from build123d import *

# Parameters (mm, degrees)
BOSS_EXTRUDE1_DEPTH     = 1.6
CUT_EXTRUDE1_DEPTH      = 56.62202801
CUT_EXTRUDE1_DEPTH_BACK = 56.62202801
SKETCH3_R               = 1.5
SKETCH4_W               = 24
SKETCH4_H               = 10
SKETCH4_W_2             = 12
BOSS_EXTRUDE2_DEPTH     = 14
SKETCH5_W               = 18
SKETCH5_H               = 61
BOSS_EXTRUDE3_DEPTH     = 13.56


with BuildPart() as part:
    # Sketch2 → Boss-Extrude1 (new body)
    with BuildSketch(Plane(origin=(0, 0, 0), x_dir=(1, 0, 0), z_dir=(0, 1, 0))):
        with BuildLine():
            Line((34, 41.5), (-34, 41.5))
            ThreePointArc((-34, 41.5), (-36.121320344, 40.621320344), (-37, 38.5))
            Line((-37, 38.5), (-37, -38.5))
            ThreePointArc((-37, -38.5), (-36.121320344, -40.621320344), (-34, -41.5))
            Line((-34, -41.5), (34, -41.5))
            ThreePointArc((34, -41.5), (36.121320344, -40.621320344), (37, -38.5))
            Line((37, -38.5), (37, 38.5))
            ThreePointArc((37, 38.5), (36.121320344, 40.621320344), (34, 41.5))
        make_face()
    extrude(amount=BOSS_EXTRUDE1_DEPTH)

    # Sketch3 → Cut-Extrude1 (cut, two sides: drawn at the far end of the back side and taken through both)
    with BuildSketch(Plane(origin=(0, 1.6, 0), x_dir=(1, 0, 0), z_dir=(0, 1, 0)).offset(-CUT_EXTRUDE1_DEPTH_BACK)):
        with Locations(Location((-33, 23.5, 0), (0, 0, 270))):
            Circle(SKETCH3_R)
        with Locations(Location((33, 23.5, 0), (0, 0, 270))):
            Circle(SKETCH3_R)
        with Locations(Location((-33, -37.5, 0), (0, 0, 270))):
            Circle(SKETCH3_R)
        with Locations(Location((33, -37.5, 0), (0, 0, 270))):
            Circle(SKETCH3_R)
    extrude(amount=CUT_EXTRUDE1_DEPTH + CUT_EXTRUDE1_DEPTH_BACK, mode=Mode.SUBTRACT)

    # Sketch4 → Boss-Extrude2 (add)
    with BuildSketch(Plane(origin=(0, 1.6, 0), x_dir=(1, 0, 0), z_dir=(0, 1, 0))):
        with Locations((-23, 36.022367187)):
            Rectangle(SKETCH4_W, SKETCH4_H)
        with Locations((-1, 36.022367187)):
            Rectangle(SKETCH4_W_2, SKETCH4_H)
        with Locations((14, 36.022367187)):
            Rectangle(SKETCH4_W_2, SKETCH4_H)
        with Locations((29, 36.022367187)):
            Rectangle(SKETCH4_W_2, SKETCH4_H)
    extrude(amount=BOSS_EXTRUDE2_DEPTH)

    # Sketch5 → Boss-Extrude3 (add)
    with BuildSketch(Plane(origin=(0, 1.6, 0), x_dir=(1, 0, 0), z_dir=(0, 1, 0))):
        with Locations((4.88, -6.5)):
            Rectangle(SKETCH5_W, SKETCH5_H)
    extrude(amount=BOSS_EXTRUDE3_DEPTH)


solid = part.part
Geometry check sheet. Reference: the model listing, model coordinates, mm. A direction names the side the tool comes from. Coordinates: 2 decimals unless noted, no trailing zeros. Order: outer loops, then holes, each group sorted by start corner. A loop starts at its lowest first (then second) coordinate and runs counter-clockwise, first axis right, second up. Notation, with made-up numbers: (14, -12.75) - (41, -12.75) arc R20 cw to (41, 5.25) - close; hole circle Ø10 at (35.25, 20.25). An arc over 180 degrees is marked (long way). Answer in a Markdown table with one row per item. Add a question column.
1) Gauge pin test, flat ends, axial feed: P1, Ø2, axis at y = 5.5, z = -5, coming from the -X side; P2, Ø7, axis at x = 5.5, y = 9, coming from the -Z side; P3, Ø1, axis at x = 11.5, y = 10, coming from the +Z side. Record the tip position at first contact, or that the pin passes through.
2) Material ranges on line 1 along X through (y, z) = (1.15, -23.5); line 2 along Z through (x, y) = (33, 0.55); line 3 along X through (y, z) = (7.25, -34), recorded low to high. Write a range as [from, to].
3) Release check for a two-part mould opening along Z. For faces 6 (the flat face through (8, 9, -36)), 7 (the flat face through (-1, 9, -31.022)), 8 (the flat face through (14, 9, -41.022)) record: +Z half, -Z half, draft (parallel to the pull), parting line (faces both ways), or undercut.
4) Cross-section at C-C, the plane z = -34.5. Record the cut outline in (x, y), then the cut area to 3 significant figures.
5) Cross-section at D-D, the plane x = 10. Record the cut outline in (y, z).
6) Cross-section at A-A, the plane y = 7.5. Record the cut outline in (x, z).
7) Cross-section at B-B, the plane x = 33. Record the cut outline in (y, z).
8) Set-up check for faces 1 (the flat face through (14, 9, -31.022)), 2 (the flat face through (5, 8, 37)), 3 (the flat face through (-1, 9, -41.022)), 4 (the flat face through (23, 9, -36)), 5 (the flat face through (13.88, 8, 7)): record each of +Z, -Z, +X, -X, +Y, -Y from which the full face is reachable in a straight line by a thin tool's end or side.
Check result:
| question | item | result |
|---|---|---|
| 1 | P1 | stops at x = -4.12 |
| 1 | P2 | stops at z = -41.02 |
| 1 | P3 | stops at z = 37 |
| 2 | line 1 | x = [-37, -34.5], [-31.5, 31.5], [34.5, 37] |
| 2 | line 2 | z = [-41.5, -25], [-22, 36], [39, 41.5] |
| 2 | line 3 | x = [-35, -11], [-7, 5], [8, 20], [23, 35] |
| 3 | face 6 | draft |
| 3 | face 7 | undercut |
| 3 | face 8 | -Z half |
| 4 | outline | (-37, 0) - (37, 0) - (37, 1.6) - (35, 1.6) - (35, 15.6) - (23, 15.6) - (23, 1.6) - (20, 1.6) - (20, 15.6) - (8, 15.6) - (8, 1.6) - (5, 1.6) - (5, 15.6) - (-7, 15.6) - (-7, 1.6) - (-11, 1.6) - (-11, 15.6) - (-35, 15.6) - (-35, 1.6) - (-37, 1.6) - close |
| 4 | area | 958 mm² |
| 5 | outline | (0, -41.5) - (1.6, -41.5) - (1.6, -41.02) - (15.6, -41.02) - (15.6, -31.02) - (1.6, -31.02) - (1.6, -24) - (15.16, -24) - (15.16, 37) - (1.6, 37) - (1.6, 41.5) - (0, 41.5) - close |
| 6 | outline | (-35, -41.02) - (-11, -41.02) - (-11, -31.02) - (-35, -31.02) - close; (-7, -41.02) - (5, -41.02) - (5, -31.02) - (-7, -31.02) - close; (-4.12, -24) - (13.88, -24) - (13.88, 37) - (-4.12, 37) - close; (8, -41.02) - (20, -41.02) - (20, -31.02) - (8, -31.02) - close; (23, -41.02) - (35, -41.02) - (35, -31.02) - (23, -31.02) - close |
| 7 | outline | (0, -41.5) - (1.6, -41.5) - (1.6, -41.02) - (15.6, -41.02) - (15.6, -31.02) - (1.6, -31.02) - (1.6, -25) - (0, -25) - close; (0, -22) - (1.6, -22) - (1.6, 36) - (0, 36) - close; (0, 39) - (1.6, 39) - (1.6, 41.5) - (0, 41.5) - close |
| 8 | face 1 | +X, -X, +Y |
| 8 | face 2 | +Z, +X, -X, +Y |
| 8 | face 3 | -Z, +X, -X, +Y |
| 8 | face 4 | +Z, -Z, +Y |
| 8 | face 5 | +Z, +X, +Y |
